```python
from build123d import *

# Parameters (mm, degrees)
SKETCH1_W             = 127
SKETCH1_H             = 77.47
BOSS_EXTRUDE1_DEPTH   = 6.35
F_8_CLEARANCE_HOLE1_D = 4.9149
FILLET1_R             = 6.35
SKETCH8_R             = 6.477
CUT_EXTRUDE1_DEPTH    = 149.899037606


with BuildPart() as part:
    # Sketch1 → Boss-Extrude1 (new body)
    with BuildSketch(Plane.XY):
        with Locations((63.5, 38.735)):
            Rectangle(SKETCH1_W, SKETCH1_H)
    extrude(amount=BOSS_EXTRUDE1_DEPTH)

    # #8 Clearance Hole1 (through all)
    with Locations(Plane.XY.offset(6.35)):
        with Locations((20.6248, 11.1125), (44.45, 11.1125), (82.55, 11.1125), (106.3752, 11.1125)):
            Hole(F_8_CLEARANCE_HOLE1_D / 2)

    # Fillet1
    fillet1_edges = [part.edges().sort_by_distance(p)[0] for p in [
        (0, 77.47, 3.175),
        (127, 77.47, 3.175),
        (127, 0, 3.175),
        (0, 0, 3.175),
    ]]
    fillet(fillet1_edges, radius=FILLET1_R)

    # Sketch8 → Cut-Extrude1 (cut, through all)
    with BuildSketch(Plane.XY.offset(6.35)):
        with Locations((63.5, 64.77)):
            Circle(SKETCH8_R)
    extrude(amount=-CUT_EXTRUDE1_DEPTH, mode=Mode.SUBTRACT)


solid = part.part
```
Work out the finished part from the listing and answer in its coordinate system (mm). Round coordinates to 2 decimals unless told otherwise and drop trailing zeros. Write each loop counter-clockwise with the first axis right and the second up, starting at its lowest first coordinate (ties: lowest second). Pieces come first, ordered by that corner, then holes.
1) A cutting plane is placed at A-A on x = 63.5. Determine the outline of the cut face in (y, z).
2) Consider probe 1 along Y at (x, z) = (82.55, 2); probe 2 along Y at (x, z) = (121, 1.25); probe 3 along X at (y, z) = (59, 0.5). Determine where each line is inside the solid, lowest interval first.
3) Determine the mould class of faces 1 (the face through (0, 38, 3)), 2 (the face through (42.18, 10.17, 3.13)), 3 (the face through (63, 0, 3)), 4 (the face through (105.241, 8.932, 3.131)) for opening direction X: pulls with the +X half, pulls with the -X half, needs draft (parallel to the pull), parting line crosses it, or undercut.
4) A cutting plane is placed at B-B on y = 60. Determine the outline of the cut face in (x, z).
5) A cutting plane is placed at C-C on z = 4.5. Determine the outline of the cut face in (x, y).
Entries:
1. outline: (0, 0) - (58.29, 0) - (58.29, 6.35) - (0, 6.35) - close; (71.25, 0) - (77.47, 0) - (77.47, 6.35) - (71.25, 6.35) - close
2. probe 1: y = 0 to 8.66, 13.57 to 77.47
2. probe 2: y = 0.01 to 77.46
2. probe 3: x = 0 to 60.56, 66.44 to 127
3. face 1: pulls with the -X half
3. face 2: undercut
3. face 3: needs draft
3. face 4: undercut
4. outline: (0, 0) - (59.12, 0) - (59.12, 6.35) - (0, 6.35) - close; (67.88, 0) - (127, 0) - (127, 6.35) - (67.88, 6.35) - close
5. outline: (0, 6.35) arc R6.35 ccw to (6.35, 0) - (120.65, 0) arc R6.35 ccw to (127, 6.35) - (127, 71.12) arc R6.35 ccw to (120.65, 77.47) - (6.35, 77.47) arc R6.35 ccw to (0, 71.12) - close; hole circle Ø4.91 at (20.62, 11.11); hole circle Ø4.91 at (44.45, 11.11); hole circle Ø12.95 at (63.5, 64.77); hole circle Ø4.91 at (82.55, 11.11); hole circle Ø4.91 at (106.38, 11.11)
